For this review, take the finished solid that the model builds, in its own axes (mm). A direction names the side the tool comes from. Coordinates: 2 decimals unless noted, no trailing zeros. Order: outer loops, then holes, each group sorted by start corner. A loop starts at its lowest first (then second) coordinate and runs counter-clockwise, first axis right, second up.
from build123d import *

# Parameters (mm, degrees)
SKETCH_1_R          = 12.5
EXTRUDE_1_DEPTH     = 1.5
SKETCH_2_R          = 11
EXTRUDE_2_DEPTH     = 4.5
SKETCH_3_R          = 5
CUT_EXTRUDE_1_DEPTH = 9
SKETCH_4_R          = 9.5
SKETCH_4_R_2        = 7
CUT_EXTRUDE_2_DEPTH = 0.5
SKETCH_5_R          = 9.5
SKETCH_5_R_2        = 7
CUT_EXTRUDE_3_DEPTH = 0.5


with BuildPart() as part:
    # 草图1 → 凸台-拉伸1 (new body)
    with BuildSketch(Plane(origin=(0, 0, 0), x_dir=(1, 0, 0), z_dir=(0, 1, 0))):
        Circle(SKETCH_1_R)
    extrude(amount=EXTRUDE_1_DEPTH)

    # 草图2 → 凸台-拉伸2 (add)
    with BuildSketch(Plane(origin=(0, 1.5, 0), x_dir=(1, 0, 0), z_dir=(0, 1, 0))):
        Circle(SKETCH_2_R)
    extrude(amount=EXTRUDE_2_DEPTH)

    # 草图3 → 切除-拉伸1 (cut)
    with BuildSketch(Plane(origin=(0, 6, 0), x_dir=(1, 0, 0), z_dir=(0, 1, 0))):
        Circle(SKETCH_3_R)
    extrude(amount=-CUT_EXTRUDE_1_DEPTH, mode=Mode.SUBTRACT)

    # 草图4 → 切除-拉伸2 (cut)
    with BuildSketch(Plane.XZ):
        Circle(SKETCH_4_R)
        Circle(SKETCH_4_R_2, mode=Mode.SUBTRACT)
    extrude(amount=-CUT_EXTRUDE_2_DEPTH, mode=Mode.SUBTRACT)

    # 草图5 → 切除-拉伸3 (cut)
    with BuildSketch(Plane(origin=(0, 6, 0), x_dir=(1, 0, 0), z_dir=(0, 1, 0))):
        Circle(SKETCH_5_R)
        Circle(SKETCH_5_R_2, mode=Mode.SUBTRACT)
    extrude(amount=-CUT_EXTRUDE_3_DEPTH, mode=Mode.SUBTRACT)


solid = part.part
1. Clearance check with flat-ended pins moving along their axes: pin 1 Ø3 at (y, z) = (2.5, -8.5) entering from -X; pin 2 Ø1.5 at (y, z) = (1, -2) entering from +X; pin 3 Ø1 at (y, z) = (3.5, 5) entering from +X. State where each tip first meets the part, or that it passes through.
Answer below:
pin 1: stops at x = -10.09
pin 2: stops at x = 12.44
pin 3: stops at x = 10.04
2. The part is to be moulded in two halves that separate along X. For faces 4 (the face through (11.923, 0.74, -3.755)), 5 (the face through (-4, 0.5, -6)), 6 (the face through (-2, 6, -5)), say which applies: +X half, -X half, draft (parallel to the pull), parting line (faces both ways), or undercut.
Answer below:
face 4: parting line
face 5: undercut
face 6: draft
3. Take a section at C-C, the plane y = 3.4. Give the boundary of the cut face in (x, z), plus the area to 3 significant figures.
Answer below:
outline: circle Ø22 at (0, 0); hole circle Ø10 at (0, 0)
area: 302 mm2
4. Take a section at A-A, the plane x = 0. Give the boundary of the cut face in (y, z), plus the area to 3 significant figures.
Answer below:
outline: (0, -12.5) - (1.5, -12.5) - (1.5, -11) - (6, -11) - (6, -9.5) - (5.5, -9.5) - (5.5, -7) - (6, -7) - (6, -5) - (0, -5) - (0, -7) - (0.5, -7) - (0.5, -9.5) - (0, -9.5) - close; (0, 5) - (6, 5) - (6, 7) - (5.5, 7) - (5.5, 9.5) - (6, 9.5) - (6, 11) - (1.5, 11) - (1.5, 12.5) - (0, 12.5) - (0, 9.5) - (0.5, 9.5) - (0.5, 7) - (0, 7) - close
area: 71.5 mm2
5. Take a section at B-B, the plane z = 0. Give the boundary of the cut face in (x, y), plus the area to 3 significant figures.
Answer below:
outline: (-12.5, 0) - (-9.5, 0) - (-9.5, 0.5) - (-7, 0.5) - (-7, 0) - (-5, 0) - (-5, 6) - (-7, 6) - (-7, 5.5) - (-9.5, 5.5) - (-9.5, 6) - (-11, 6) - (-11, 1.5) - (-12.5, 1.5) - close; (5, 0) - (7, 0) - (7, 0.5) - (9.5, 0.5) - (9.5, 0) - (12.5, 0) - (12.5, 1.5) - (11, 1.5) - (11, 6) - (9.5, 6) - (9.5, 5.5) - (7, 5.5) - (7, 6) - (5, 6) - close
area: 71.5 mm2
6. Machinability: for faces 1 (the face through (5, 1.5, 10)), 2 (the face through (6.466, 0.246, -2.681)), 3 (the face through (-1.08, 3.04, 4.88)), which of the approach directions +Z, -Z, +X, -X, +Y, -Y give a long, thin tool a straight path to every point of the face, cutting with its end or side? Answer none if there is none.
Answer below:
face 1: +Y
face 2: -Y
face 3: +Y, -Y
7. To check wall thickness, follow L1, parallel to X at y = 5.95, z = 0; L2, parallel to X at y = 2.15, z = 0; L3, parallel to Y at x = 9.25, z = 7.75. State the ranges of each line that lie inside material, in increasing order.
Answer below:
L1: x = -11 to -9.5, -7 to -5, 5 to 7, 9.5 to 11
L2: x = -11 to -5, 5 to 11
L3: y = 0 to 1.5
8. Take a section at D-D, the plane x = -10.5. Give the boundary of the cut face in (y, z).
Answer below:
outline: (0, -6.78) - (1.5, -6.78) - (1.5, -3.28) - (6, -3.28) - (6, 3.28) - (1.5, 3.28) - (1.5, 6.78) - (0, 6.78) - close
